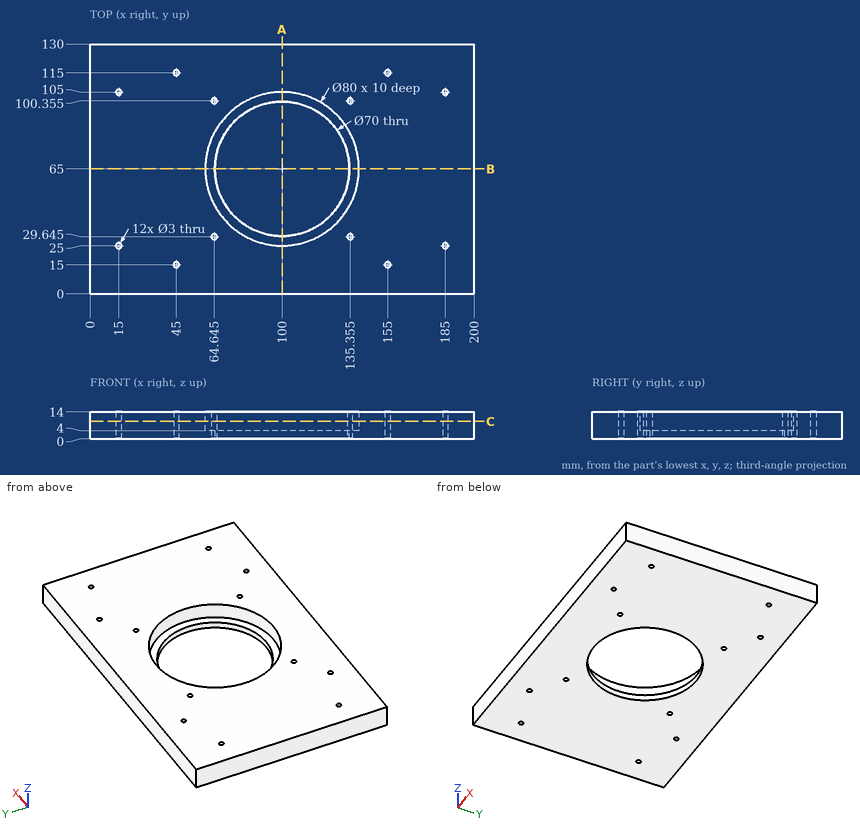
Could you check a few things on this drawing? It's one solid part, dimensions in mm from its lowest x, y, z. Coordinates: 2 decimals unless noted, no trailing zeros. Write each loop counter-clockwise with the first axis right and the second up, starting at its lowest first coordinate (ties: lowest second). Pieces come first, ordered by that corner, then holes. Notation, with made-up numbers: (-14, 13.5) - (18, 13.5) arc R20 cw to (18, 18.5) - close; hole circle Ø9 at (25.25, 68.25). An arc over 180 degrees is marked (long way). Put each result on its own line as item: value. Start each with the question number.
Q1. I'm going to push a flat-ended pin straight in: P1, Ø2.5, axis at x = 155, y = 115, coming from the +Z side. Where does the tip first touch, or does it pass through?
Q2. I want a section at A-A on x = 100. Write out the boundary of the cut face in (y, z).
Q3. Please list where these lines run through material, in increasing order: L1, parallel to Y at x = 155, z = 6; L2, parallel to Y at x = 15, z = 7.5; L3, parallel to X at y = 115, z = 3.
Q4. I want a section at C-C on z = 9. Count the separate pieces of the cut face and the enclosed holes in it, plus the area to 3 significant figures.
Q5. I want a section at B-B on y = 65. Write out the boundary of the cut face in (x, z).
Checks:
1. P1: through
2. outline: (0, 0) - (30, 0) - (30, 4) - (25, 4) - (25, 14) - (0, 14) - close; (100, 0) - (130, 0) - (130, 14) - (105, 14) - (105, 4) - (100, 4) - close
3. L1: 0 to 13.5, 16.5 to 113.5, 116.5 to 130
3. L2: 0 to 23.5, 26.5 to 103.5, 106.5 to 130
3. L3: 0 to 43.5, 46.5 to 153.5, 156.5 to 200
4. separate pieces: 1
4. enclosed holes: 13
4. area: 20,900 mm²
5. outline: (0, 0) - (65, 0) - (65, 4) - (60, 4) - (60, 14) - (0, 14) - close; (135, 0) - (200, 0) - (200, 14) - (140, 14) - (140, 4) - (135, 4) - close
